Can you work these out from the model? Positions are in its coordinate system, mm. Face numbers are marked on the shaded views. A direction names the side the tool comes from. Give positions to 0.01 mm unless a question says otherwise; leave off trailing zeros. Order: outer loops, then holes, each group sorted by start corner. A loop starts at its lowest first (then second) coordinate and runs counter-clockwise, first axis right, second up.
Autodesk Inventor part; units mm, degrees
ref_plane "YZ Plane" through (0, 0, 0) normal (1, 0, 0) x (0, 1, 0)
ref_plane "XZ Plane" through (0, 0, 0) normal (0, 1, 0) x (-1, 0, 0)
ref_plane "XY Plane" through (0, 0, 0) normal (0, 0, 1) x (1, 0, 0)
sketch "Szkic1" plane through (0, 0, 0) normal (0, 1, 0) x (-1, 0, 0)
  circle A0 centre (0, -143.2209) radius 25
  line L0 (25, -143.2209) -> (25, -78.2209)
  line L1 (25, -78.2209) -> (57.3466, -78.2209)
  line L2 (57.3466, -78.2209) -> (57.3466, -33.2209)
  line L3 (57.3466, -33.2209) -> (47.3466, -33.2209)
  line L4 (47.3466, -33.2209) -> (47.3466, -68.2209)
  line L5 (47.3466, -68.2209) -> (15, -68.2209)
  line L6 (15, -68.2209) -> (15, -108.2209)
  line L7 (15, -108.2209) -> (0, -108.2209)
  line L8 (0, -108.2209) -> (0, 0)
  line L9 (-25, -143.2209) -> (-25, -78.2209)
  line L10 (-25, -78.2209) -> (-57.3466, -78.2209)
  line L11 (-57.3466, -78.2209) -> (-57.3466, -33.2209)
  line L12 (-57.3466, -33.2209) -> (-47.3466, -33.2209)
  line L13 (-47.3466, -33.2209) -> (-47.3466, -68.2209)
  line L14 (-47.3466, -68.2209) -> (-15, -68.2209)
  line L15 (-15, -68.2209) -> (-15, -108.2209)
  line L16 (-15, -108.2209) -> (0, -108.2209)
  point P0 (7.5, -108.2209)
  point P1 (52.3466, -33.2209)
  dimension "d0" = 50
  dimension "d1" = 35
  dimension "d2" = 65
  dimension "d3" = 10
  dimension "d4" = 45
  dimension "d5" = 15
  dimension "d6" = 10
  dimension "d7" = 10
extrude "Wyciągnięcie proste1" add sketch "Szkic1" along normal blind 40 contours A0 L9 L10 L11 L12 L13 L14 L15 L16 L7 L6 L5 L4 L3 L2 L1 L0
sketch "Szkic2" plane through (0, 40, 0) normal (0, 1, 0) x (1, 0, 0)
  point P0 (0, 0)
sketch "Szkic3" plane through (0, 40, 0) normal (0, 1, 0) x (1, 0, 0)
  circle A0 centre (0, 143.2209) radius 25
  point P0 (0, 0)
extrude "Wyciągnięcie proste2" add sketch "Szkic3" along normal blind 30 and the other way blind 50
sketch "Szkic4" plane through (0, 70, -143.2209) normal (0, 1, 0) x (1, 0, 0)
  circle A0 centre (0, 0) radius 17.5
  point P0 (0, -143.2209)
  dimension "d14" = 35
extrude "Wyciągnięcie proste3" add sketch "Szkic4" along normal blind 16
sketch "Szkic5" plane through (0, 86, -143.2209) normal (0, 1, 0) x (1, 0, 0)
  point P0 (0, -143.2209)
  point P1 (0, 0)
hole "Otwór1" at (0, 86, -143.2209) direction (0, -1, 0) diameter 20 end through all
sketch "Szkic6" plane through (57.3466, 0, -33.2209) normal (1, 0, 0) x (0, 0, -1)
  line L0 (0, 0) -> (0, 40)
  circle A0 centre (35, 20.3911) radius 35
  line L1 (0, 0) -> (0, 40)
  line L2 (35, 40) -> (0, 40)
  line L3 (6.0088, 40) -> (0, 40)
  line L4 (35, 0) -> (0, 0)
  line L5 (0, 40) -> (0, 0)
  line L6 (0, 0) -> (6.5535, 0)
  point P0 (-33.2209, 0)
  point P1 (0, 20.3911)
  dimension "d24" = 70
extrude "Wyciągnięcie proste4" cut sketch "Szkic6" against normal through all contours L0 A0 L4 | L0 L2 A0
sketch "Szkic7" plane through (57.3466, 0, -78.2209) normal (1, 0, 0) x (0, 0, -1)
  line L0 (-38.4465, 0) -> (0, 0)
  arc A0 (-38.9912, 40) -> (-38.4465, 0) centre (-10, 20.3911) ccw
  point P0 (-78.2209, 0)
  point P1 (-25, 20)
  dimension "d27" = 20
  dimension "d28" = 15
hole "Otwór2" at (57.3466, 20, -53.2209) direction (-1, 0, 0) diameter 12 end through all
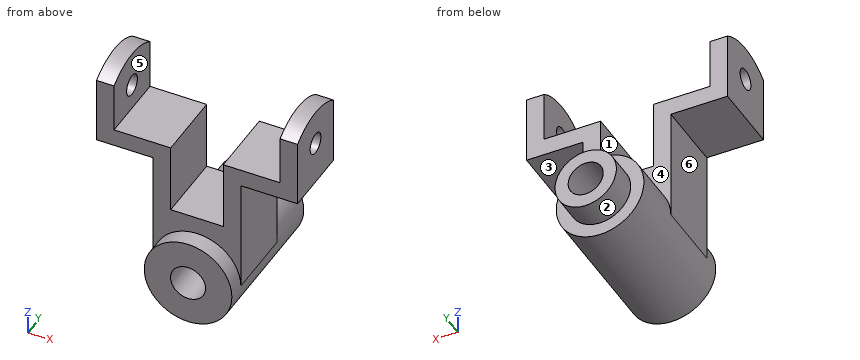
1) Suppose I cut it at A-A (z = -63). Please give me the cut outline in (x, y).
2) Suppose I cut it at D-D (y = 77). Please give me the cut outline in (x, z).
3) Suppose I cut it at B-B (y = 20). Please give me the cut outline in (x, z), and give its area (3 significant figures).
4) I'm going to push flat-ended pins straight in: pin 1 Ø14 at (y, z) = (20, -53.22) entering from -X; pin 2 Ø5 at (y, z) = (66.5, -147.5) entering from +X; pin 3 Ø9.5 at (x, y) = (41.5, 12) entering from -Z; pin 4 Ø3 at (y, z) = (20, -91) entering from -X. Where does each tip first touch, or does it pass through?
5) If I drill on line 1 (Z direction, x = 0, y = 62.5); line 2 (Z direction, x = -52.25, y = 20); line 3 (X direction, y = 23.5, z = -106.5), over which ranges is the centre line in solid material (lowest first)?
6) Which directions (+Z, -Z, +X, -X, +Y, -Y) give clear straight access to the entire face, cutting with the end or side of a thin tool? Please do the marked faces 1, 2 and 3.
7) Suppose I cut it at C-C (x = 0). Please give me the cut outline in (y, z), and give its area (3 significant figures).
8) We'd pull the mould along X, two halves only. Please class the marked faces 4, 5 and 6: +X half, -X half, draft (parallel to the pull), parting line (faces both ways), or undercut.
Results:
1. outline: (-57.35, 0) - (-47.35, 0) - (-47.35, 40) - (-57.35, 40) - close; (47.35, 0) - (57.35, 0) - (57.35, 40) - (47.35, 40) - close
2. outline: circle Ø35 at (0, -143.22); hole circle Ø20 at (0, -143.22)
3. outline: (-57.35, -78.22) - (-25, -78.22) - (-25, -143.22) arc R25 ccw to (25, -143.22) - (25, -78.22) - (57.35, -78.22) - (57.35, -59.22) - (47.35, -59.22) - (47.35, -68.22) - (15, -68.22) - (15, -108.22) - (-15, -108.22) - (-15, -68.22) - (-47.35, -68.22) - (-47.35, -59.22) - (-57.35, -59.22) - close; (-57.35, -47.22) - (-47.35, -47.22) - (-47.35, -33.22) - (-57.35, -33.22) - close; (47.35, -47.22) - (57.35, -47.22) - (57.35, -33.22) - (47.35, -33.22) - close; hole circle Ø20 at (0, -143.22)
3. area: 4,320 mm2
4. pin 1: stops at x = -57.35
4. pin 2: stops at x = 24.94
4. pin 3: stops at z = -78.22
4. pin 4: stops at x = -25
5. line 1: z = -168.22 to -153.22, -133.22 to -118.22
5. line 2: z = -78.22 to -59.22, -47.22 to -33.22
5. line 3: x = -25 to -15, 15 to 25
6. face 1: +Z, +Y, -Y
6. face 2: +Y
6. face 3: -Z, +X, +Y, -Y
7. outline: (-10, -168.22) - (70, -168.22) - (70, -160.72) - (86, -160.72) - (86, -153.22) - (-10, -153.22) - close; (-10, -133.22) - (86, -133.22) - (86, -125.72) - (70, -125.72) - (70, -118.22) - (40, -118.22) - (40, -108.22) - (0, -108.22) - (0, -118.22) - (-10, -118.22) - close
7. area: 3,040 mm2
8. face 4: draft
8. face 5: undercut
8. face 6: -X half
